Geometry check sheet. Reference: the model listing, model coordinates, mm. Round coordinates to 2 decimals unless told otherwise and drop trailing zeros. Order: outer loops, then holes, each group sorted by start corner. A loop starts at its lowest first (then second) coordinate and runs counter-clockwise, first axis right, second up. Notation, with made-up numbers: (-5.5, 72.25) - (3.5, 72.25) arc R18 cw to (3.5, 97.25) - close; hole circle Ø3 at (59, -37). An arc over 180 degrees is marked (long way). Write each question's results on one line, items separated by ' | '.
```python
from build123d import *

# Parameters (mm, degrees)
SKETCH1_W           = 140
SKETCH1_H           = 170
BOSS_EXTRUDE1_DEPTH = 5
CHAMFER1_SIZE       = 15
SKETCH2_R           = 9.75
CUT_EXTRUDE1_DEPTH  = 5
SKETCH3_R           = 2.75
CUT_EXTRUDE2_DEPTH  = 40
SKETCH4_R           = 1.75
CUT_EXTRUDE3_DEPTH  = 6


with BuildPart() as part:
    # Sketch1 → Boss-Extrude1 (new body)
    with BuildSketch(Plane(origin=(0, 0, 0), x_dir=(1, 0, 0), z_dir=(0, 1, 0))):
        Rectangle(SKETCH1_W, SKETCH1_H)
    extrude(amount=BOSS_EXTRUDE1_DEPTH)

    # Chamfer1
    chamfer1_edges = [part.edges().sort_by_distance(p)[0] for p in [
        (-70, 2.5, -85),
        (70, 2.5, -85),
        (70, 2.5, 85),
        (-70, 2.5, 85),
    ]]
    chamfer(chamfer1_edges, length=CHAMFER1_SIZE)

    # Sketch2 → Cut-Extrude1 (cut)
    with BuildSketch(Plane(origin=(0, 5, 0), x_dir=(1, 0, 0), z_dir=(0, 1, 0))):
        Circle(SKETCH2_R)
    extrude(amount=-CUT_EXTRUDE1_DEPTH, mode=Mode.SUBTRACT)

    # Sketch3 → Cut-Extrude2 (cut)
    with BuildSketch(Plane(origin=(0, 5, 0), x_dir=(1, 0, 0), z_dir=(0, 1, 0))):
        with Locations((0, -67.5)):
            Circle(SKETCH3_R)
        with Locations((0, 67.5)):
            Circle(SKETCH3_R)
    extrude(amount=-CUT_EXTRUDE2_DEPTH, mode=Mode.SUBTRACT)

    # Sketch4 → Cut-Extrude3 (cut, through all)
    with BuildSketch(Plane(origin=(0, 5, 0), x_dir=(1, 0, 0), z_dir=(0, 1, 0))):
        with Locations((-21, 0)):
            Circle(SKETCH4_R)
        with Locations((21, 0)):
            Circle(SKETCH4_R)
    extrude(amount=-CUT_EXTRUDE3_DEPTH, mode=Mode.SUBTRACT)


solid = part.part
```
(1) Material ranges on line 1 (X direction, y = 3.95, z = 0); line 2 (Z direction, x = 0, y = 3.75); line 3 (X direction, y = 2.5, z = -67.5), recorded low to high.
Answers follow:
line 1: -70 to -22.75, -19.25 to -9.75, 9.75 to 19.25, 22.75 to 70 | line 2: -85 to -70.25, -64.75 to -9.75, 9.75 to 64.75, 70.25 to 85 | line 3: -70 to -2.75, 2.75 to 70
(2) Depth check by flat-ended pin: pin 1 Ø5.5 at (x, z) = (21, 0) entering from -Y. Enter the tip coordinate at first touch or a pass-through.
Answers follow:
pin 1: y = 0
(3) Section check C-C (x = 0). Record the cut outline in (y, z), then the cut area to 4 significant figures.
Answers follow:
outline: (0, -85) - (5, -85) - (5, -70.25) - (0, -70.25) - close; (0, -64.75) - (5, -64.75) - (5, -9.75) - (0, -9.75) - close; (0, 9.75) - (5, 9.75) - (5, 64.75) - (0, 64.75) - close; (0, 70.25) - (5, 70.25) - (5, 85) - (0, 85) - close | area: 697.5 mm²
(4) Section check B-B (y = 4.1). Record the cut outline in (x, z), then the cut area to 3 significant figures.
Answers follow:
outline: (-70, -70) - (-55, -85) - (55, -85) - (70, -70) - (70, 70) - (55, 85) - (-55, 85) - (-70, 70) - close; hole circle Ø3.5 at (-21, 0); hole circle Ø19.5 at (0, 0); hole circle Ø5.5 at (0, -67.5); hole circle Ø5.5 at (0, 67.5); hole circle Ø3.5 at (21, 0) | area: 23,000 mm²
(5) Section check A-A (z = -67.5). Record the cut outline in (x, y).
Answers follow:
outline: (-70, 0) - (-2.75, 0) - (-2.75, 5) - (-70, 5) - close; (2.75, 0) - (70, 0) - (70, 5) - (2.75, 5) - close
